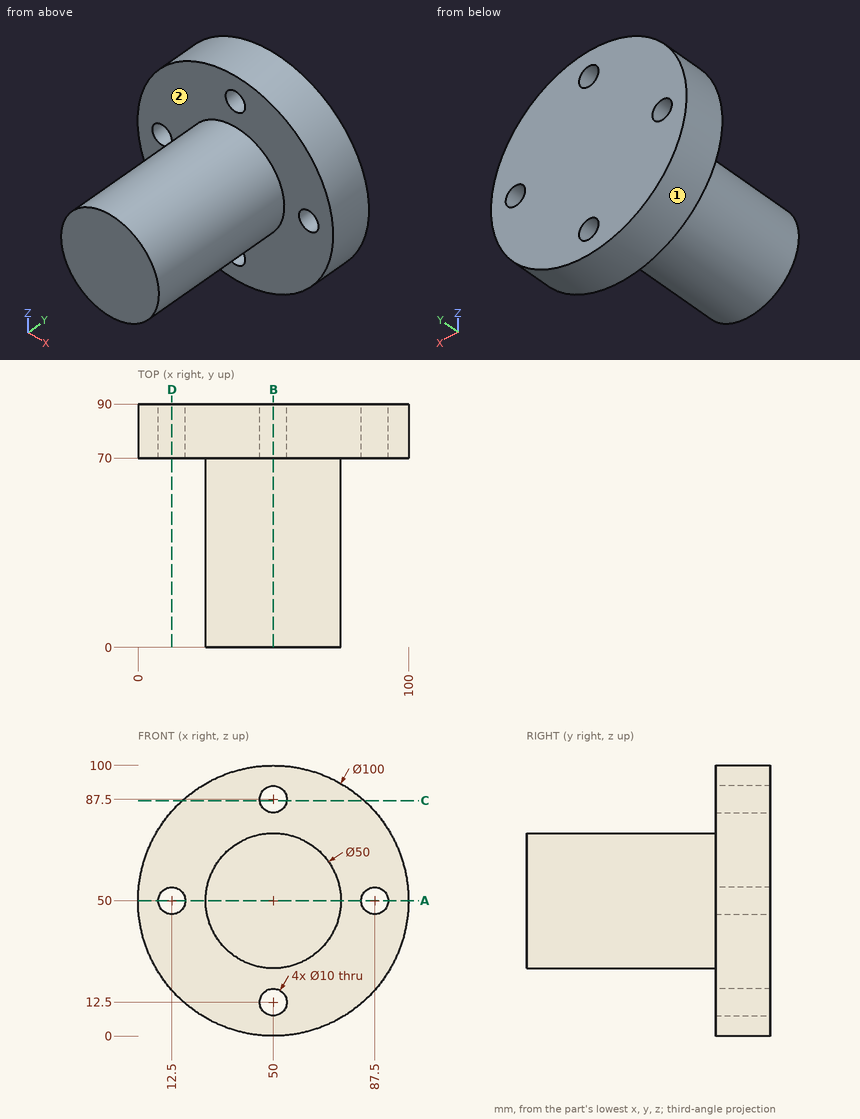
Source: three-view drawing plus pictorial views. Frame: mm from the lowest corner of the part. A direction names the side the tool comes from. Give positions to 0.01 mm unless a question says otherwise; leave off trailing zeros. Write each loop counter-clockwise with the first axis right and the second up, starting at its lowest first coordinate (ties: lowest second). Pieces come first, ordered by that corner, then holes. Notation, with made-up numbers: (7.25, 44.25) - (66.25, 44.25) arc R3 ccw to (66.25, 49.25) - close; hole circle Ø3 at (65.25, 8). An arc over 180 degrees is marked (long way). Write item = value, one per line. Start each with the question number.
Q1. Material intervals for probe 1 along X at (y, z) = (79, 51); probe 2 along Z at (x, y) = (12, 77), sorted ascending.
Q2. Reachability of the marked faces 1 and 2 from +Z, -Z, +X, -X, +Y, -Y: full face, straight path, thin tool, end or side. Return the list, or none.
Q3. Cut plane D-D, the plane x = 12.5. Return loops of the section in (y, z), then the cut area to 3 significant figures.
Q4. Cut plane B-B, the plane x = 50. Return loops of the section in (y, z).
Q5. Cut plane C-C, the plane z = 87. Return loops of the section in (x, y), then the cut area to 3 significant figures.
Q6. Cut plane A-A, the plane z = 50. Return loops of the section in (x, y).
Q7. Pin query (flat end, axial travel): pin 1 Ø9 at (x, z) = (12.5, 50) entering from -Y; pin 2 Ø12 at (y, z) = (65.5, 12) entering from +X; pin 3 Ø16 at (x, z) = (87.5, 50) entering from -Y; pin 4 Ø1.5 at (y, z) = (12, 72) entering from +X. Return the tip coordinate at first contact, or that it passes through.
Computed values:
q1.probe_1 = 0.01 to 7.6, 17.4 to 82.6, 92.4 to 99.99
q1.probe_2 = 17.5 to 45.03, 54.97 to 82.5
q2.face_1 = +Y, -Y
q2.face_2 = -Y
q3.outline = (70, 16.93) - (90, 16.93) - (90, 45) - (70, 45) - close; (70, 55) - (90, 55) - (90, 83.07) - (70, 83.07) - close
q3.area = 1,120 mm²
q4.outline = (0, 25) - (70, 25) - (70, 17.5) - (90, 17.5) - (90, 82.5) - (70, 82.5) - (70, 75) - (0, 75) - close; (70, 0) - (90, 0) - (90, 7.5) - (70, 7.5) - close; (70, 92.5) - (90, 92.5) - (90, 100) - (70, 100) - close
q5.outline = (16.37, 70) - (45.03, 70) - (45.03, 90) - (16.37, 90) - close; (54.97, 70) - (83.63, 70) - (83.63, 90) - (54.97, 90) - close
q5.area = 1,150 mm²
q6.outline = (0, 70) - (7.5, 70) - (7.5, 90) - (0, 90) - close; (17.5, 70) - (25, 70) - (25, 0) - (75, 0) - (75, 70) - (82.5, 70) - (82.5, 90) - (17.5, 90) - close; (92.5, 70) - (100, 70) - (100, 90) - (92.5, 90) - close
q7.pin_1 = through
q7.pin_2 = 86.63
q7.pin_3 = 70
q7.pin_4 = 63.17
